Design review of the part built by this model. Coordinates are the model's own, in mm. A direction names the side the tool comes from. Coordinates: 2 decimals unless noted, no trailing zeros. Loops run counter-clockwise (first coordinate to the right, second up) from the corner with the lowest first, then second, coordinate; pieces in that order, holes last. Notation, with made-up numbers: (41.25, 88) -> (66.25, 88) arc R12 cw to (66.25, 110) -> close; hole circle Ø9 at (-16, 56.25). An arc over 180 degrees is marked (long way). Answer as a JSON object with one key per item and string values.
```python
from build123d import *

# Parameters (mm, degrees)
SKETCH2_R             = 4.5
SKETCH2_R_2           = 2.5
BOSS_EXTRUDE2_DEPTH   = 7.5
BOSS_EXTRUDE2_2_DEPTH = 7.5
BOSS_EXTRUDE2_3_DEPTH = 7.5
BOSS_EXTRUDE2_4_DEPTH = 7.5
SKETCH2_10_R          = 4.5
SKETCH2_10_R_2        = 2.5
BOSS_EXTRUDE4_DEPTH   = 2.5


with BuildPart() as part:
    # Sketch2 → Boss-Extrude2 (new body)
    with BuildSketch(Plane(origin=(0, 0, 0), x_dir=(1, 0, 0), z_dir=(0, 1, 0))):
        with Locations(Location((95, 8, 0), (0, 0, 270))):
            Circle(SKETCH2_R)
        with Locations(Location((95, 8, 0), (0, 0, 270))):
            Circle(SKETCH2_R_2, mode=Mode.SUBTRACT)
    extrude(amount=BOSS_EXTRUDE2_DEPTH)



with BuildPart() as body_2:
    # Sketch2 → Boss-Extrude2 2 (new body)
    with BuildSketch(Plane(origin=(0, 0, 0), x_dir=(1, 0, 0), z_dir=(0, 1, 0))):
        with Locations(Location((95, 62, 0), (0, 0, 270))):
            Circle(SKETCH2_R)
        with Locations(Location((95, 62, 0), (0, 0, 270))):
            Circle(SKETCH2_R_2, mode=Mode.SUBTRACT)
    extrude(amount=BOSS_EXTRUDE2_2_DEPTH)


with BuildPart() as body_3:
    # Sketch2 → Boss-Extrude2 3 (new body)
    with BuildSketch(Plane(origin=(0, 0, 0), x_dir=(1, 0, 0), z_dir=(0, 1, 0))):
        with Locations(Location((8, 62, 0), (0, 0, 270))):
            Circle(SKETCH2_R)
        with Locations(Location((8, 62, 0), (0, 0, 270))):
            Circle(SKETCH2_R_2, mode=Mode.SUBTRACT)
    extrude(amount=BOSS_EXTRUDE2_3_DEPTH)


with BuildPart() as body_4:
    # Sketch2 → Boss-Extrude2 4 (new body)
    with BuildSketch(Plane(origin=(0, 0, 0), x_dir=(1, 0, 0), z_dir=(0, 1, 0))):
        with Locations(Location((8, 8, 0), (0, 0, 270))):
            Circle(SKETCH2_R)
        with Locations(Location((8, 8, 0), (0, 0, 270))):
            Circle(SKETCH2_R_2, mode=Mode.SUBTRACT)
    extrude(amount=BOSS_EXTRUDE2_4_DEPTH)


with BuildPart() as part_1:
    add(part.part)

    add(body_2.part)  # Boss-Extrude4 merges body 2

    add(body_3.part)  # Boss-Extrude4 merges body 3

    add(body_4.part)  # Boss-Extrude4 merges body 4
    # Sketch2_10 → Boss-Extrude4 (add)
    # profile 1 of 5: a face of its own
    with BuildSketch(Plane(origin=(0, 0, 0), x_dir=(1, 0, 0), z_dir=(0, 1, 0))):
        with BuildLine():
            Line((3, 2.7), (100, 2.7))
            ThreePointArc((100, 2.7), (100.212132034, 2.787867966), (100.3, 3))
            Line((100.3, 3), (100.3, 67))
            ThreePointArc((100.3, 67), (100.212132034, 67.212132034), (100, 67.3))
            Line((100, 67.3), (3, 67.3))
            ThreePointArc((3, 67.3), (2.787867966, 67.212132034), (2.7, 67))
            Line((2.7, 67), (2.7, 3))
            ThreePointArc((2.7, 3), (2.787867966, 2.787867966), (3, 2.7))
        make_face()
        with Locations(Location((8, 62, 0), (0, 0, 270))):
            Circle(SKETCH2_10_R, mode=Mode.SUBTRACT)
        with Locations(Location((95, 8, 0), (0, 0, 270))):
            Circle(SKETCH2_10_R, mode=Mode.SUBTRACT)
        with Locations(Location((95, 62, 0), (0, 0, 270))):
            Circle(SKETCH2_10_R, mode=Mode.SUBTRACT)
        with Locations(Location((8, 8, 0), (0, 0, 270))):
            Circle(SKETCH2_10_R, mode=Mode.SUBTRACT)
    # profile 2 of 5: a face of its own
    with BuildSketch(Plane(origin=(0, 0, 0), x_dir=(1, 0, 0), z_dir=(0, 1, 0))):
        with Locations(Location((8, 8, 0), (0, 0, 270))):
            Circle(SKETCH2_10_R_2)
    # profile 3 of 5: a face of its own
    with BuildSketch(Plane(origin=(0, 0, 0), x_dir=(1, 0, 0), z_dir=(0, 1, 0))):
        with Locations(Location((8, 62, 0), (0, 0, 270))):
            Circle(SKETCH2_10_R_2)
    # profile 4 of 5: a face of its own
    with BuildSketch(Plane(origin=(0, 0, 0), x_dir=(1, 0, 0), z_dir=(0, 1, 0))):
        with Locations(Location((95, 8, 0), (0, 0, 270))):
            Circle(SKETCH2_10_R_2)
    # profile 5 of 5: a face of its own
    with BuildSketch(Plane(origin=(0, 0, 0), x_dir=(1, 0, 0), z_dir=(0, 1, 0))):
        with Locations(Location((95, 62, 0), (0, 0, 270))):
            Circle(SKETCH2_10_R_2)
    extrude(amount=BOSS_EXTRUDE4_DEPTH)


solid = part_1.part
```
1) Add section B-B, the plane z = -8. Give the boundary of the cut face in (x, y).
Completed:
{"outline": "(2.7, 0) -> (100.3, 0) -> (100.3, 2.5) -> (99.5, 2.5) -> (99.5, 7.5) -> (97.5, 7.5) -> (97.5, 2.5) -> (92.5, 2.5) -> (92.5, 7.5) -> (90.5, 7.5) -> (90.5, 2.5) -> (12.5, 2.5) -> (12.5, 7.5) -> (10.5, 7.5) -> (10.5, 2.5) -> (5.5, 2.5) -> (5.5, 7.5) -> (3.5, 7.5) -> (3.5, 2.5) -> (2.7, 2.5) -> close"}
2) For faces 1 (the cylindrical face through (5.56, 4.96, -8.54)), 2 (the flat face through (52, 1, -67.3)), list the 3-axis set-ups (+Z, -Z, +X, -X, +Y, -Y) from which the entire face can be reached by the end or side of a thin tool; tool diameter is ignored.
Completed:
{"face 1": "+Y", "face 2": "-Z, +X, -X, +Y, -Y"}
3) Add section C-C, the plane x = 8. Give the boundary of the cut face in (y, z), and give its area (4 significant figures).
Completed:
{"outline": "(0, -67.3) -> (2.5, -67.3) -> (2.5, -66.5) -> (7.5, -66.5) -> (7.5, -64.5) -> (2.5, -64.5) -> (2.5, -59.5) -> (7.5, -59.5) -> (7.5, -57.5) -> (2.5, -57.5) -> (2.5, -12.5) -> (7.5, -12.5) -> (7.5, -10.5) -> (2.5, -10.5) -> (2.5, -5.5) -> (7.5, -5.5) -> (7.5, -3.5) -> (2.5, -3.5) -> (2.5, -2.7) -> (0, -2.7) -> close", "area": "201.5 mm²"}
4) The part is to be moulded in two halves that separate along X. For faces 3 (the cylindrical face through (97.48, 4.96, -62.33)), 4 (the flat face through (2.7, 1, -35)), 5 (the flat face through (93, 7.5, -60)), say which applies: pulls with the +X half, pulls with the -X half, needs draft (parallel to the pull), parting line crosses it, or undercut.
Completed:
{"face 3": "undercut", "face 4": "pulls with the -X half", "face 5": "needs draft"}
5) Add section A-A, the plane y = 4. Give the boundary of the cut face in (x, z).
Completed:
{"outline": "circle Ø9 at (8, -62); circle Ø9 at (8, -8); circle Ø9 at (95, -62); circle Ø9 at (95, -8); hole circle Ø5 at (8, -62); hole circle Ø5 at (8, -8); hole circle Ø5 at (95, -62); hole circle Ø5 at (95, -8)"}
6) Clearance check with flat-ended pins moving along their axes: pin 1 Ø3 at (y, z) = (4.5, -26.5) entering from -X; pin 2 Ø1.5 at (x, z) = (96, -62) entering from +Y. State where each tip first meets the part, or that it passes through.
Completed:
{"pin 1": "through", "pin 2": "y = 2.5"}
7) Wall thickness on probe 1 along X at (y, z) = (6.1, -62); probe 2 along Y at (x, z) = (82.5, -45.5); probe 3 along X at (y, z) = (6, -7.5): over which ranges is each line inside the solid? List them lowest first.
Completed:
{"probe 1": "3.5 to 5.5, 10.5 to 12.5, 90.5 to 92.5, 97.5 to 99.5", "probe 2": "0 to 2.5", "probe 3": "3.53 to 5.55, 10.45 to 12.47, 90.53 to 92.55, 97.45 to 99.47"}
8) Add section D-D, the plane x = 91.5. Give the boundary of the cut face in (y, z), and give its area (3 significant figures).
Completed:
{"outline": "(0, -67.3) -> (2.5, -67.3) -> (2.5, -64.83) -> (7.5, -64.83) -> (7.5, -59.17) -> (2.5, -59.17) -> (2.5, -10.83) -> (7.5, -10.83) -> (7.5, -5.17) -> (2.5, -5.17) -> (2.5, -2.7) -> (0, -2.7) -> close", "area": "218 mm²"}
